```python
from build123d import *

# Parameters (mm, degrees)
F1_DEPTH = 258.572
F3_DEPTH = 12.7
F5_DEPTH = 12.7


with BuildPart() as f1:
    # F0 (on Top) → F1 (new body)
    with BuildSketch(Plane.XY):
        with BuildLine():
            ThreePointArc((12.7, 6.35), (10.840128, 10.840128), (6.35, 12.7))
            Line((6.35, 12.7), (-6.35, 12.7))
            ThreePointArc((-6.35, 12.7), (-10.840128, 10.840128), (-12.7, 6.35))
            Line((-12.7, 6.35), (-12.7, -6.35))
            ThreePointArc((-12.7, -6.35), (-10.840128, -10.840128), (-6.35, -12.7))
            Line((-6.35, -12.7), (6.35, -12.7))
            ThreePointArc((6.35, -12.7), (10.840128, -10.840128), (12.7, -6.35))
            Line((12.7, -6.35), (12.7, 6.35))
        make_face()
    extrude(amount=F1_DEPTH)

    # F2 (on Right) → F3 (cut, symmetric)
    with BuildSketch(Plane.YZ):
        Polygon((-17.71266, 0), (12.69978, 0), (-17.71266, 2.660744), align=None)
    extrude(amount=F3_DEPTH, both=True, mode=Mode.SUBTRACT)

    # F4 (on Right) → F5 (cut, symmetric)
    with BuildSketch(Plane.YZ):
        Polygon((-13.926481, 256.242485), (12.7, 258.572), (-13.926481, 258.572), align=None)
    extrude(amount=F5_DEPTH, both=True, mode=Mode.SUBTRACT)


solid = f1.part
```
Check sheet for the modelled part. Datum: model origin and axes. Units: mm. Round coordinates to 2 decimals unless told otherwise and drop trailing zeros. Loops run counter-clockwise (first coordinate to the right, second up) from the corner with the lowest first, then second, coordinate; pieces in that order, holes last. Notation, with made-up numbers: (-36.5, 35) -> (19.5, 35) arc R15 cw to (19.5, 56) -> close; hole circle Ø6 at (67, -25). An arc over 180 degrees is marked (long way). Write item = value, one per line. Start each with the question number.
1) Sectioned sample at B-B, the plane x = -9. Record the cut outline in (y, z).
2) Thickness scan on probe 1 along X at (y, z) = (6.5, 185.5); probe 2 along Z at (x, y) = (6, -1.5). Record the ranges inside material, lowest first.
3) Gauge pin test, flat ends, axial feed: pin 1 Ø1 at (y, z) = (9.5, 94) entering from -X; pin 2 Ø6 at (x, y) = (-8, -6.5) entering from +Z; pin 3 Ø1 at (x, y) = (-1.5, -6) entering from +Z. Record the tip position at first contact, or that the pin passes through.
4) Sectioned sample at A-A, the plane z = 126. Record the cut outline in (x, y).
5) Sectioned sample at C-C, the plane y = 10.5. Record the cut outline in (x, z), plus the area to 3 significant figures.
6) Release check for a two-part mould opening along Y. For faces 1 (the flat face through (12.7, 0, 127)), 2 (the cylindrical face through (-10.79, 10.89, 127.48)), 3 (the cylindrical face through (-10.89, -10.79, 127.5)) record: released by +Y, released by -Y, zero draft, split by the parting line, or undercut.
Results are:
q1.outline = (-12.12, 2.17) -> (12.12, 0.05) -> (12.12, 258.52) -> (-12.12, 256.4) -> close
q2.probe_1 = -12.7 to 12.7
q2.probe_2 = 1.24 to 257.33
q3.pin_1 = -12.12
q3.pin_2 = 257.15
q3.pin_3 = 256.98
q4.outline = (-12.7, -6.35) arc R6.35 ccw to (-6.35, -12.7) -> (6.35, -12.7) arc R6.35 ccw to (12.7, -6.35) -> (12.7, 6.35) arc R6.35 ccw to (6.35, 12.7) -> (-6.35, 12.7) arc R6.35 ccw to (-12.7, 6.35) -> close
q5.outline = (-11.16, 0.19) -> (11.16, 0.19) -> (11.16, 258.38) -> (-11.16, 258.38) -> close
q5.area = 5,760 mm^2
q6.face_1 = zero draft
q6.face_2 = released by +Y
q6.face_3 = released by -Y
